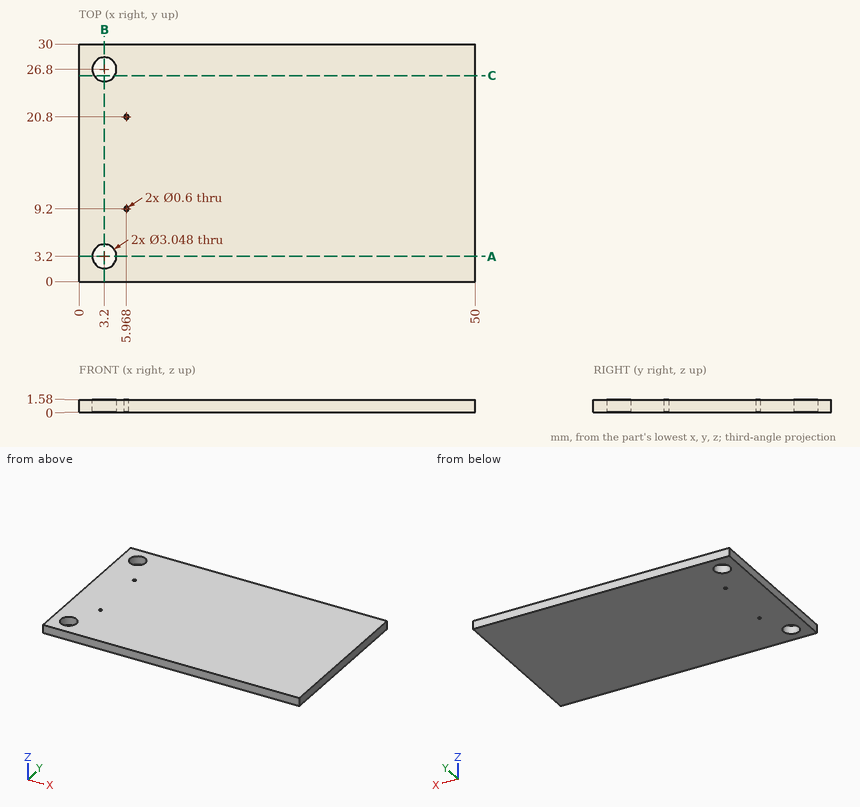
Geometry: see drawing. Coordinates: mm, zero at the bounding-box minimum. Give positions to 0.01 mm unless a question says otherwise; leave off trailing zeros. Order: outer loops, then holes, each group sorted by start corner. A loop starts at its lowest first (then second) coordinate and runs counter-clockwise, first axis right, second up. Notation, with made-up numbers: (42.25, -23) -> (95.25, -23) arc R27 cw to (95.25, -7) -> close; hole circle Ø7 at (-29.75, 75). An arc over 180 degrees is marked (long way). Write each question's results on one line, items separated by ' | '. Start each with the question number.
1) Section A-A (y = 3.2). Return loops of the section in (x, z).
2) Section C-C (y = 26). Return loops of the section in (x, z), then the cut area to 3 significant figures.
3) First-contact query: pin 1 (2.5 mm diameter, centred on x = 3.2, y = 26.8, fed in from -Z). Flat tip, straight axial feed; report the tip coordinate or a pass-through.
4) Section B-B (x = 3.2). Return loops of the section in (y, z).
5) Line query: line 1 (X direction, y = 20.8, z = 0.75); line 2 (X direction, y = 26.8, z = 0.85). Output: solid intervals per line, ascending. Write a range as from..to.
Calculated:
1) outline: (0, 0) -> (1.68, 0) -> (1.68, 1.58) -> (0, 1.58) -> close; (4.72, 0) -> (50, 0) -> (50, 1.58) -> (4.72, 1.58) -> close
2) outline: (0, 0) -> (1.9, 0) -> (1.9, 1.58) -> (0, 1.58) -> close; (4.5, 0) -> (50, 0) -> (50, 1.58) -> (4.5, 1.58) -> close | area: 74.9 mm2
3) pin 1: through
4) outline: (0, 0) -> (1.68, 0) -> (1.68, 1.58) -> (0, 1.58) -> close; (4.72, 0) -> (25.28, 0) -> (25.28, 1.58) -> (4.72, 1.58) -> close; (28.32, 0) -> (30, 0) -> (30, 1.58) -> (28.32, 1.58) -> close
5) line 1: 0..5.67, 6.27..50 | line 2: 0..1.68, 4.72..50
